Can you work these out from the model? Positions are in its coordinate system, mm. A direction names the side the tool comes from. Give positions to 0.01 mm unless a question says otherwise; leave off trailing zeros. Order: outer loops, then holes, each group sorted by start corner. A loop starts at its lowest first (then second) coordinate and runs counter-clockwise, first axis right, second up. Notation, with made-up numbers: (13.5, 72.25) - (51.5, 72.25) arc R17 cw to (51.5, 82.25) - close; hole circle Ø11 at (-5.75, -9.75). An arc over 180 degrees is marked (long way). Write each question's results on one line, items separated by ' | '. Start each with the question number.
from build123d import *

# Parameters (mm, degrees)
F0_W     = 39
F0_H     = 20
F1_DEPTH = 30
F2_W     = 31.625382
F2_H     = 11.189356
F3_DEPTH = 39.8


with BuildPart() as f1:
    # F0 (on Front) → F1 (new body)
    with BuildSketch(Plane.XZ):
        Rectangle(F0_W, F0_H)
    extrude(amount=F1_DEPTH)

    # F2 (on face) → F3 (join)
    with BuildSketch(Plane.XZ.offset(30)):
        with Locations((-0.341064, 0.578394)):
            Rectangle(F2_W, F2_H)
    extrude(amount=-F3_DEPTH)


solid = f1.part
Q1. If we section it at D-D (z = -7.5): Please give me the cut outline in (x, y), plus the area to 3 significant figures.
Q2. If we section it at C-C (y = 5): Please give me the cut outline in (x, z).
Q3. If we section it at A-A (z = 2.5): Please give me the cut outline in (x, y).
Q4. Will these pins go through, and if not, where does the flat tip stop? P1, Ø3, axis at y = 3.5, z = -2, coming from the +X side; P2, Ø6, axis at x = 5, y = 5, coming from the +Z side; P3, Ø5, axis at y = 7, z = 2.5, coming from the -X side.
Q5. If we section it at B-B (x = 12): Please give me the cut outline in (y, z).
Q6. If I drill on probe 1 along X at (y, z) = (4, -1.5); probe 2 along Y at (x, z) = (1.5, 7.25); probe 3 along Z at (x, y) = (2.5, 1), over which ranges is the centre line in solid material (lowest first)? Write a range as from..to.
Q7. Thinking about a two-plate mould opening in Y: for faces 1 (the flat face through (-1, 9.8, 1)), 2 (the flat face through (0, -15, 10)), 3 (the flat face through (0, -30, 0)), which applies, released by +Y, released by -Y, zero draft, split by the parting line, or undercut?
Q8. Which directions (+Z, -Z, +X, -X, +Y, -Y) give clear straight access to the entire face, cutting with the end or side of a thin tool? Please do faces 4 (the flat face through (-1, 5, -5.016)), 5 (the flat face through (15.472, 5, 1)), 6 (the flat face through (-1, 5, 6.173)), 7 (the flat face through (-16.154, 5, 1)).
Findings below:
1) outline: (-19.5, -30) - (19.5, -30) - (19.5, 0) - (-19.5, 0) - close | area: 1,170 mm2
2) outline: (-16.15, -5.02) - (15.47, -5.02) - (15.47, 6.17) - (-16.15, 6.17) - close
3) outline: (-19.5, -30) - (19.5, -30) - (19.5, 0) - (15.47, 0) - (15.47, 9.8) - (-16.15, 9.8) - (-16.15, 0) - (-19.5, 0) - close
4) P1: stops at x = 15.47 | P2: stops at z = 6.17 | P3: stops at x = -16.15
5) outline: (-30, -10) - (0, -10) - (0, -5.02) - (9.8, -5.02) - (9.8, 6.17) - (0, 6.17) - (0, 10) - (-30, 10) - close
6) probe 1: x = -16.15..15.47 | probe 2: y = -30..0 | probe 3: z = -5.02..6.17
7) face 1: released by +Y | face 2: zero draft | face 3: released by -Y
8) face 4: -Z, +X, -X, +Y | face 5: +Z, -Z, +X, +Y | face 6: +Z, +X, -X, +Y | face 7: +Z, -Z, -X, +Y
